Geometry: see drawing. Coordinates: mm, zero at the bounding-box minimum. A direction names the side the tool comes from. Coordinates: 2 decimals unless noted, no trailing zeros. Write each loop counter-clockwise with the first axis right and the second up, starting at its lowest first coordinate (ties: lowest second). Pieces come first, ordered by that corner, then holes. Notation, with made-up numbers: (54.5, 36) - (110.5, 36) arc R28 cw to (110.5, 63) - close; hole circle Ø3 at (-27.75, 11.5). An arc over 180 degrees is marked (long way). Use a Markdown table: item, result. Add a question column.
Q1. Set-up query: the marked faces 1, 2 and 3. Return all of +Z, -Z, +X, -X, +Y, -Y with unobstructed straight access to the full face (end or side cutting, diameter ignored); none if empty.
Q2. Section query C-C (z = 36.5). Return the cut outline in (x, y), then the cut area to 3 significant figures.
Q3. Mould query, pull axis Z, two halves, no side actions, for the marked faces 4, 5 and 6. Classes: released by +Z, released by -Z, zero draft, split by the parting line, or undercut.
Q4. Section query B-B (x = 10). Return the cut outline in (y, z), then the cut area to 3 significant figures.
Q5. Pin query (flat end, axial travel): P1, Ø1, axis at x = 21, z = 24, coming from the -Y side; P2, Ø10, axis at x = 9.5, y = 12.5, coming from the -Z side; P3, Ø1.5, axis at y = 17, z = 8, coming from the +X side. Return the tip coordinate at first contact, or that it passes through.
Q6. Section query A-A (x = 15.5). Return the cut outline in (y, z).
Q7. Section query D-D (y = 54). Return the cut outline in (x, z).
Q8. Material intervals for probe 1 along X at (y, z) = (26.5, 30); probe 2 along Y at (x, z) = (29.5, 37.5); probe 3 along Z at (x, y) = (35.5, 30.5) (1 decimal), sorted ascending. Write a range as from..to.
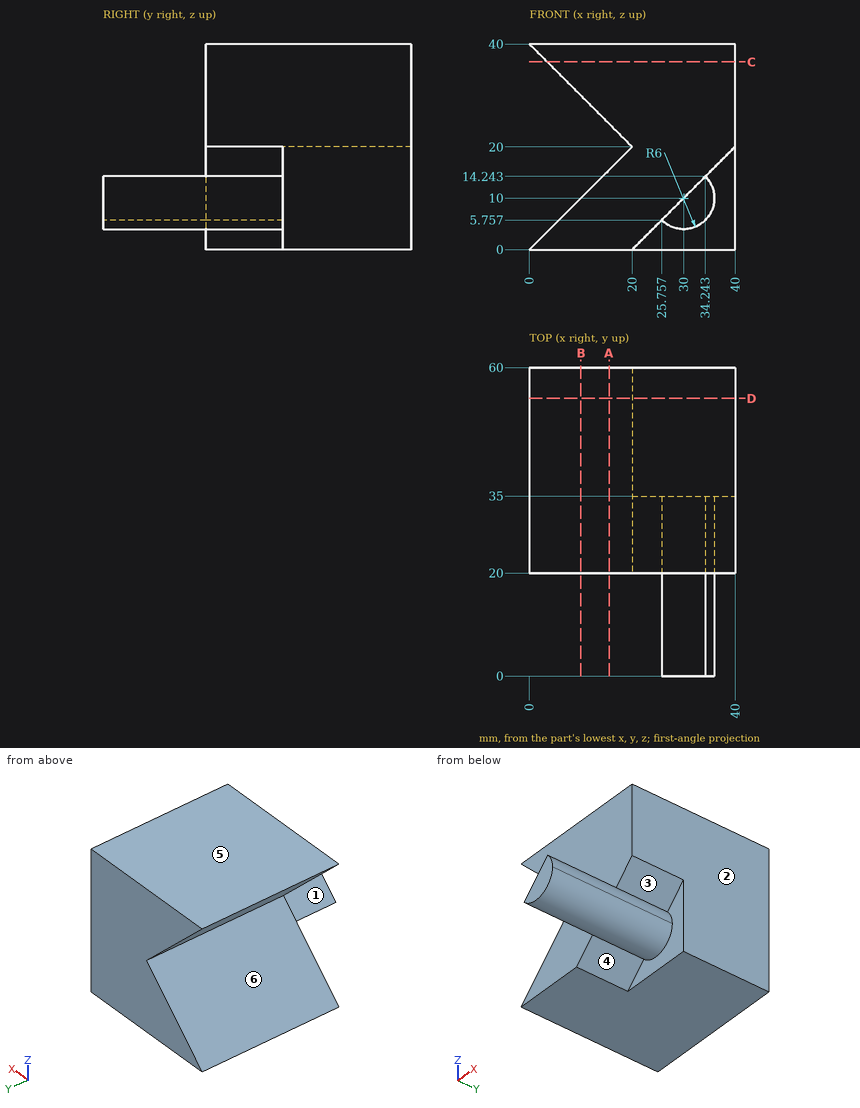
Values follow:
| question | item | result |
|---|---|---|
| 1 | face 1 | +Z, -X, -Y |
| 1 | face 2 | +Z, -Z, +X, +Y, -Y |
| 1 | face 3 | +X, -Y |
| 2 | outline | (3.5, 20) - (40, 20) - (40, 60) - (3.5, 60) - close |
| 2 | area | 1,460 mm2 |
| 3 | face 4 | released by -Z |
| 3 | face 5 | released by +Z |
| 3 | face 6 | undercut |
| 4 | outline | (20, 0) - (60, 0) - (60, 10) - (20, 10) - close; (20, 30) - (60, 30) - (60, 40) - (20, 40) - close |
| 4 | area | 800 mm2 |
| 5 | P1 | y = 20 |
| 5 | P2 | through |
| 5 | P3 | x = 35.87 |
| 6 | outline | (20, 0) - (60, 0) - (60, 15.5) - (20, 15.5) - close; (20, 24.5) - (60, 24.5) - (60, 40) - (20, 40) - close |
| 7 | outline | (0, 0) - (40, 0) - (40, 40) - (0, 40) - (20, 20) - close |
| 8 | probe 1 | 10..40 |
| 8 | probe 2 | 20..60 |
| 8 | probe 3 | 7.6..12.4, 15.5..40 |
